Verification items for the finished model (mm, model axes). A direction names the side the tool comes from. Coordinates: 2 decimals unless noted, no trailing zeros. Write each loop counter-clockwise with the first axis right and the second up, starting at its lowest first coordinate (ties: lowest second). Pieces come first, ordered by that corner, then holes. Notation, with made-up numbers: M 84,14 L 102,14 A13 ccw 102,29 Z; hole C -8.75,-27 d3. An arc over 180 degrees is marked long. One line per item, written item: value.
```python
from build123d import *

# Parameters (mm, degrees)
SKETCH1_R           = 2
SKETCH1_W           = 12.7
SKETCH1_H           = 50.8
BOSS_EXTRUDE3_DEPTH = 6.35


with BuildPart() as part:
    # Sketch1 → Boss-Extrude3 (new body)
    with BuildSketch(Plane(origin=(0, 0, 0), x_dir=(1, 0, 0), z_dir=(0, 1, 0))):
        with BuildLine():
            ThreePointArc((32.240681933, -66.10056535), (0, -48.302004425), (-32.240681933, -66.10056535))
            ThreePointArc((-32.240681933, -66.10056535), (-33.11372382, -66.748004461), (-34.194833578, -66.63583839))
            ThreePointArc((-34.194833578, -66.63583839), (0, 74.897407173), (34.194833578, -66.63583839))
            ThreePointArc((34.194833578, -66.63583839), (33.11372382, -66.748004461), (32.240681933, -66.10056535))
        make_face()
        with Locations((-51.004123727, -33.414457974)):
            Circle(SKETCH1_R, mode=Mode.SUBTRACT)
        with Locations((7.824123727, -33.623956053)):
            Circle(SKETCH1_R, mode=Mode.SUBTRACT)
        with Locations((51.004123727, -33.623956053)):
            Circle(SKETCH1_R, mode=Mode.SUBTRACT)
        with Locations((51.004123727, 34.956043947)):
            Circle(SKETCH1_R, mode=Mode.SUBTRACT)
        with Locations((-7.824123727, 35.165542026)):
            Circle(SKETCH1_R, mode=Mode.SUBTRACT)
        with Locations((-7.824123727, -33.414457974)):
            Circle(SKETCH1_R, mode=Mode.SUBTRACT)
        with Locations((-51.004123727, 35.165542026)):
            Circle(SKETCH1_R, mode=Mode.SUBTRACT)
        with Locations((-46.663733983, -40.081231883)):
            Circle(SKETCH1_R, mode=Mode.SUBTRACT)
        with Locations((46.663733983, -40.081231883)):
            Circle(SKETCH1_R, mode=Mode.SUBTRACT)
        with Locations((46.663733983, 40.081231883)):
            Circle(SKETCH1_R, mode=Mode.SUBTRACT)
        with Locations((-46.663733983, 40.081231883)):
            Circle(SKETCH1_R, mode=Mode.SUBTRACT)
        with Locations((7.824123727, 34.956043947)):
            Circle(SKETCH1_R, mode=Mode.SUBTRACT)
        with Locations((61.164123727, 0)):
            Rectangle(SKETCH1_W, SKETCH1_H, mode=Mode.SUBTRACT)
        with Locations((-61.164123727, 0)):
            Rectangle(SKETCH1_W, SKETCH1_H, mode=Mode.SUBTRACT)
    extrude(amount=BOSS_EXTRUDE3_DEPTH)


solid = part.part
```
Item 1: Scan lines: line 1 (X direction, y = 1, z = 0.5); line 2 (Z direction, x = 50, y = 3); line 3 (X direction, y = 1.75, z = 11.5). Record each from-to range of solid material in increasing order.
The answers:
line 1: x = -74.9 to -67.51, -54.81 to 54.81, 67.51 to 74.9
line 2: z = -55.76 to -36.69, -33.23 to 31.89, 35.35 to 55.76
line 3: x = -74.01 to -67.51, -54.81 to 54.81, 67.51 to 74.01
Item 2: Go/stop test with flat-tipped pins: P1, Ø1.9, axis at x = 60.5, y = 3, coming from the -Z side; P2, Ø4.5, axis at x = 46.66, z = 40.08, coming from the +Y side; P3, Ø2.5, axis at x = -51, z = 33.41, coming from the -Y side; P4, Ø3, axis at x = 33.5, y = 2, coming from the -Z side. Record where each tip stops, or that it passes through.
The answers:
P1: stops at z = -45.42
P2: stops at y = 6.35
P3: passes through
P4: stops at z = -67.72
Item 3: Cross-section at D-D, the plane x = 0. Enter the section's corners in (y, z), and give its area (3 significant figures).
The answers:
outline: M 0,-74.9 L 6.35,-74.9 L 6.35,48.3 L 0,48.3 Z
area: 782 mm²
Item 4: Cross-section at B-B, the plane x = 58.5. Enter the section's corners in (y, z).
The answers:
outline: M 0,-46.77 L 6.35,-46.77 L 6.35,-25.4 L 0,-25.4 Z; M 0,25.4 L 6.35,25.4 L 6.35,46.77 L 0,46.77 Z
Item 5: Draft check along Z on faces 1 (the face through (1, 6.35, -5)), 2 (the face through (-48.66, 3.13, 39.99)). Enter one of: released by +Z, released by -Z, zero draft, split by the parting line, or undercut.
The answers:
face 1: zero draft
face 2: undercut
Item 6: Cross-section at A-A, the plane z = 0. Enter the section's corners in (x, y), and give its area (3 significant figures).
The answers:
outline: M -74.9,0 L -67.51,0 L -67.51,6.35 L -74.9,6.35 Z; M -54.81,0 L 54.81,0 L 54.81,6.35 L -54.81,6.35 Z; M 67.51,0 L 74.9,0 L 74.9,6.35 L 67.51,6.35 Z
area: 790 mm²
Item 7: Access from +Z, -Z, +X, -X, +Y, -Y to the whole of each face (thin tool, end or side, straight path). Record for faces 3 (the face through (54.814, 3, 0)), 4 (the face through (1, 0, -5)).
The answers:
face 3: +Y, -Y
face 4: +Z, -Z, +X, -X, -Y
Item 8: Cross-section at C-C, the plane y = 2. Give the number of separate pieces and of enclosed holes in the cut face, and give its area (3 significant figures).
The answers:
separate pieces: 1
enclosed holes: 14
area: 15,000 mm²
